Verification items for the finished model (mm, model axes). Coordinates: 2 decimals unless noted, no trailing zeros. Order: outer loops, then holes, each group sorted by start corner. A loop starts at its lowest first (then second) coordinate and runs counter-clockwise, first axis right, second up.
Q1. Depth check by flat-ended pin: P1, Ø12, axis at x = -223.5, y = -22, coming from the +Z side. Enter the tip coordinate at first touch or a pass-through.
Q2. Cross-section at B-B, the plane x = -25. Record the boundary of the cut face in (y, z).
Q3. Thickness scan on line 1 (X direction, y = -12, z = -25.5); line 2 (X direction, y = -23.5, z = -17). Record the ranges inside material, lowest first.
Q4. Cross-section at A-A, the plane y = -20.75. Record the boundary of the cut face in (x, z).
Q5. Cross-section at C-C, the plane z = -29. Record the boundary of the cut face in (x, y).
from build123d import *

# Parameters (mm, degrees)
F1_DEPTH = 25


with BuildPart() as f1:
    # F0 (on Front) → F1 (new body)
    with BuildSketch(Plane.XZ):
        with BuildLine():
            Line((-16.161165, -16.161165), (0, 0))
            Line((0, 0), (-475, 0))
            Line((-475, 0), (-458.838835, -16.161165))
            ThreePointArc((-458.838835, -16.161165), (-445.216457, -13.451506), (-437.5, -25))
            ThreePointArc((-437.5, -25), (-438.451506, -29.783543), (-441.161165, -33.838835))
            Line((-441.161165, -33.838835), (-425, -50))
            Line((-425, -50), (-50, -50))
            Line((-50, -50), (-33.838835, -33.838835))
            ThreePointArc((-33.838835, -33.838835), (-33.838835, -16.161165), (-16.161165, -16.161165))
        make_face()
        with BuildLine():
            Line((0, -50), (0, 0))
            Line((0, 0), (-16.161165, -16.161165))
            ThreePointArc((-16.161165, -16.161165), (-13.451506, -20.216457), (-12.5, -25))
            ThreePointArc((-12.5, -25), (-20.216457, -36.548494), (-33.838835, -33.838835))
            Line((-33.838835, -33.838835), (-50, -50))
            Line((-50, -50), (0, -50))
        make_face()
        with BuildLine():
            Line((-458.838835, -16.161165), (-475, 0))
            Line((-475, 0), (-475, -50))
            Line((-475, -50), (-425, -50))
            Line((-425, -50), (-441.161165, -33.838835))
            ThreePointArc((-441.161165, -33.838835), (-458.838835, -33.838835), (-458.838835, -16.161165))
        make_face()
    extrude(amount=F1_DEPTH)


solid = f1.part
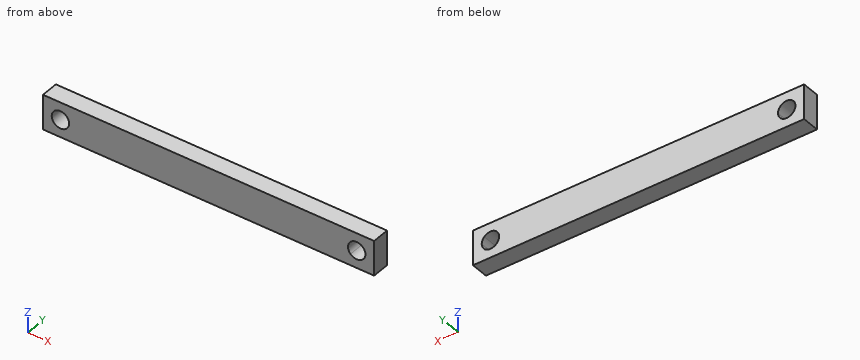
Check values:
1. P1: stops at z = 0
2. outline: (-25, -50) - (0, -50) - (0, -37.5) - (-25, -37.5) - close; (-25, -12.5) - (0, -12.5) - (0, 0) - (-25, 0) - close
3. line 1: x = -475 to -462.49, -437.51 to -37.49, -12.51 to 0
3. line 2: x = -475 to -459.6, -440.4 to -34.6, -15.4 to 0
4. outline: (-475, -50) - (0, -50) - (0, 0) - (-475, 0) - close; hole (-441.16, -33.84) arc R12.5 ccw to (-437.5, -25) arc R12.5 ccw (long way) to start; hole (-16.16, -16.16) arc R12.5 ccw (long way) to (-12.5, -25) arc R12.5 ccw to start
5. outline: (-475, -25) - (-461.84, -25) - (-461.84, 0) - (-475, 0) - close; (-438.16, -25) - (-36.84, -25) - (-36.84, 0) - (-438.16, 0) - close; (-13.16, -25) - (0, -25) - (0, 0) - (-13.16, 0) - close
